Answer from the drawing. Dimensions are ordinates in mm from the lowest x, y and z of the part. A direction names the side the tool comes from. Round coordinates to 2 decimals unless told otherwise and drop trailing zeros. Loops run counter-clockwise (first coordinate to the right, second up) from the corner with the lowest first, then second, coordinate; pieces in that order, holes last. Notation, with made-up numbers: M -28.75,-11.75 L -11.75,-11.75 A14 ccw -11.75,12.25 Z; hole C -15,44 d3. An arc over 180 degrees is marked long. Write each question's results on one line, items separated by ' | '.
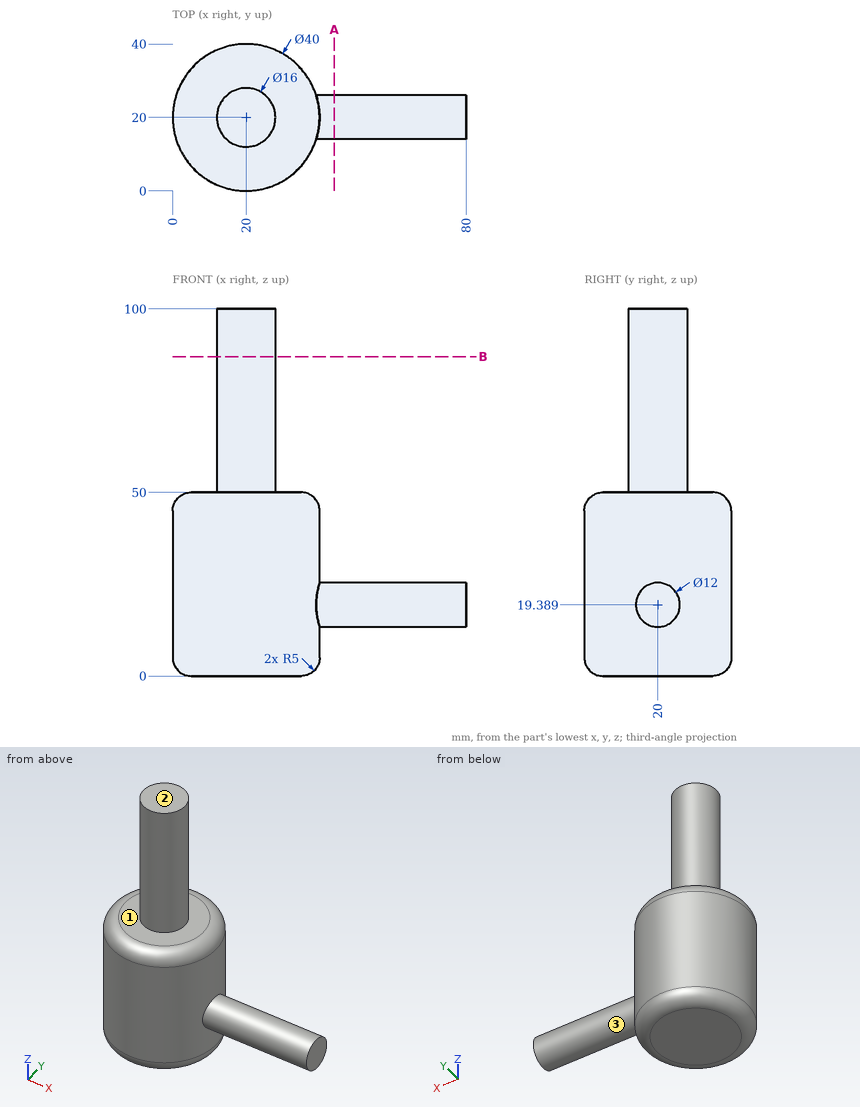
1. Find section A-A, the plane x = 44. Give the vertices of the cut face in (y, z).
Completed:
outline: C 20,19.39 d12
2. Find the intervals of material crossed by L1, parallel to Z at x = 18, y = 33; L2, parallel to Z at x = 37.5, y = 13 (1 decimal); L3, parallel to X at y = 26, z = 64.5, in increasing order.
Completed:
L1: z = 0 to 50 | L2: z = 1.8 to 48.2 | L3: x = 14.71 to 25.29
3. Find section B-B, the plane z = 87. Give the vertices of the cut face in (x, y), then the cut area to 3 significant figures.
Completed:
outline: C 20,20 d16 | area: 201 mm2
4. Which of the six approach directions +Z, -Z, +X, -X, +Y, -Y give full straight-line access (tool end or side, diameter ignored) to the marked faces 1, 2 and 3?
Completed:
face 1: +Z | face 2: +Z, +X, -X, +Y, -Y | face 3: +X
5. Given P1, Ø10, axis at y = 9, z = 36.5, coming from the -X side; P2, Ø10, axis at x = 13.5, z = 62, coming from the +Y side; P3, Ø10, axis at x = 55, y = 20.5, coming from the +Z side, each flat-ended and moving along its own axis, determine where each tip first touches the part or whether it passes through.
Completed:
P1: stops at x = 0.92 | P2: stops at y = 27.86 | P3: stops at z = 25.39
